from build123d import *

# Parameters (mm, degrees)
SKETCH_1_W          = 30
SKETCH_1_H          = 30
SKETCH_1_R          = 1.55
EXTRUDE_1_DEPTH     = 10
SKETCH_2_R          = 3.5
CUT_EXTRUDE_1_DEPTH = 3
SKETCH_3_W          = 6
SKETCH_3_H          = 15
EXTRUDE_3_DEPTH     = 3
SKETCH_5_W          = 1.5
SKETCH_5_H          = 0.7
CUT_EXTRUDE_3_DEPTH = 36


with BuildPart() as part:
    # 草图1 → 凸台-拉伸1 (new body)
    with BuildSketch(Plane(origin=(0, 0, 0), x_dir=(1, 0, 0), z_dir=(0, 1, 0))):
        Rectangle(SKETCH_1_W, SKETCH_1_H)
        with Locations(Location((-5, 5, 0), (0, 0, 270))):
            Circle(SKETCH_1_R, mode=Mode.SUBTRACT)
        with Locations(Location((5, 5, 0), (0, 0, 270))):
            Circle(SKETCH_1_R, mode=Mode.SUBTRACT)
        with Locations(Location((5, -5, 0), (0, 0, 270))):
            Circle(SKETCH_1_R, mode=Mode.SUBTRACT)
        with Locations(Location((-5, -5, 0), (0, 0, 270))):
            Circle(SKETCH_1_R, mode=Mode.SUBTRACT)
    extrude(amount=EXTRUDE_1_DEPTH)

    # 草图2 → 切除-拉伸1 (cut)
    with BuildSketch(Plane.XZ):
        with Locations(Location((-5, 5, 0), (0, 0, 270))):
            Circle(SKETCH_2_R)
        with Locations(Location((5, 5, 0), (0, 0, 270))):
            Circle(SKETCH_2_R)
        with Locations(Location((5, -5, 0), (0, 0, 270))):
            Circle(SKETCH_2_R)
        with Locations(Location((-5, -5, 0), (0, 0, 270))):
            Circle(SKETCH_2_R)
    extrude(amount=-CUT_EXTRUDE_1_DEPTH, mode=Mode.SUBTRACT)

    # 草图3 → 凸台-拉伸3 (add)
    with BuildSketch(Plane.XZ):
        with Locations((-12, 0)):
            Rectangle(SKETCH_3_W, SKETCH_3_H)
        with Locations((12, 0)):
            Rectangle(SKETCH_3_W, SKETCH_3_H)
    extrude(amount=EXTRUDE_3_DEPTH)

    # 草图5 → 切除-拉伸3 (cut, through all)
    with BuildSketch(Plane.ZY.offset(15)):
        with Locations((-6.75, -0.35)):
            Rectangle(SKETCH_5_W, SKETCH_5_H)
        with Locations((6.75, -0.35)):
            Rectangle(SKETCH_5_W, SKETCH_5_H)
    extrude(amount=-CUT_EXTRUDE_3_DEPTH, mode=Mode.SUBTRACT)


solid = part.part
Input: part model. Units: mm. Frame: model coordinates. A direction names the side the tool comes from. Coordinates: 2 decimals unless noted, no trailing zeros. Loops run counter-clockwise (first coordinate to the right, second up) from the corner with the lowest first, then second, coordinate; pieces in that order, holes last.
(1) Section D-D on x = 10.25. Return the cut outline in (y, z).
(2) First-contact query: pin 1 Ø2 at (x, z) = (-5.5, -3.5) entering from -Y; pin 2 Ø1.5 at (x, z) = (8, 7.5) entering from -Y; pin 3 Ø1.8 at (x, y) = (11.5, -2) entering from -Z. Flat tips, straight axial feed; report the tip coordinate or a pass-through.
(3) Section C-C on z = -5. Return the cut outline in (x, y), then the cut area to 3 significant figures.
(4) Material intervals for probe 1 along Z at (x, y) = (-5, 5); probe 2 along X at (y, z) = (2.4, -5), sorted ascending.
(5) Pull-direction query (Z, two-part tool) for faces 1 (the face through (-12, -2, 7.5)), 2 (the face through (15, 3, 0)), 3 (the face through (-6.341, 1.479, -8.233)); classes: released by +Z, released by -Z, zero draft, split by the parting line, or undercut.
(6) Section A-A on x = 5. Return the cut outline in (y, z), then the cut area to 3 significant figures.
(7) Section B-B on y = 8.75. Return the cut outline in (x, z).
(8) Set-up query: faces 4 (the face through (3, 3, 4)), 5 (the face through (-9, -1, 0)), 6 (the face through (12, -2, -7.5)). Return all of +Z, -Z, +X, -X, +Y, -Y with unobstructed straight access to the full face (end or side cutting, diameter ignored); none if empty.
Data:
1. outline: (-3, -7.5) - (-0.7, -7.5) - (-0.7, -6) - (0, -6) - (0, -15) - (10, -15) - (10, 15) - (0, 15) - (0, 6) - (-0.7, 6) - (-0.7, 7.5) - (-3, 7.5) - close
2. pin 1: stops at y = 3
2. pin 2: stops at y = 0
2. pin 3: stops at z = -7.5
3. outline: (-15, -3) - (-9, -3) - (-9, 0) - (-8.5, 0) - (-8.5, 3) - (-6.55, 3) - (-6.55, 10) - (-15, 10) - close; (-3.45, 3) - (-1.5, 3) - (-1.5, 0) - (1.5, 0) - (1.5, 3) - (3.45, 3) - (3.45, 10) - (-3.45, 10) - close; (6.55, 3) - (8.5, 3) - (8.5, 0) - (9, 0) - (9, -3) - (15, -3) - (15, 10) - (6.55, 10) - close
3. area: 251 mm2
4. probe 1: z = -15 to -6.55, -3.45 to 3.45, 6.55 to 15
4. probe 2: x = -15 to -8.5, -1.5 to 1.5, 8.5 to 15
5. face 1: released by +Z
5. face 2: zero draft
5. face 3: undercut
6. outline: (0, -15) - (10, -15) - (10, -6.55) - (3, -6.55) - (3, -8.5) - (0, -8.5) - close; (0, -1.5) - (3, -1.5) - (3, -3.45) - (10, -3.45) - (10, 3.45) - (3, 3.45) - (3, 1.5) - (0, 1.5) - close; (0, 8.5) - (3, 8.5) - (3, 6.55) - (10, 6.55) - (10, 15) - (0, 15) - close
6. area: 215 mm2
7. outline: (-15, -15) - (15, -15) - (15, 15) - (-15, 15) - close; hole circle Ø3.1 at (-5, -5); hole circle Ø3.1 at (-5, 5); hole circle Ø3.1 at (5, -5); hole circle Ø3.1 at (5, 5)
8. face 4: -Y
8. face 5: +Z, -Z, -Y
8. face 6: -Z, +X, -X, -Y
